Can you work these out from the model? Positions are in its coordinate system, mm. Round coordinates to 2 decimals unless told otherwise and drop trailing zeros. Loops run counter-clockwise (first coordinate to the right, second up) from the corner with the lowest first, then second, coordinate; pieces in that order, holes last.
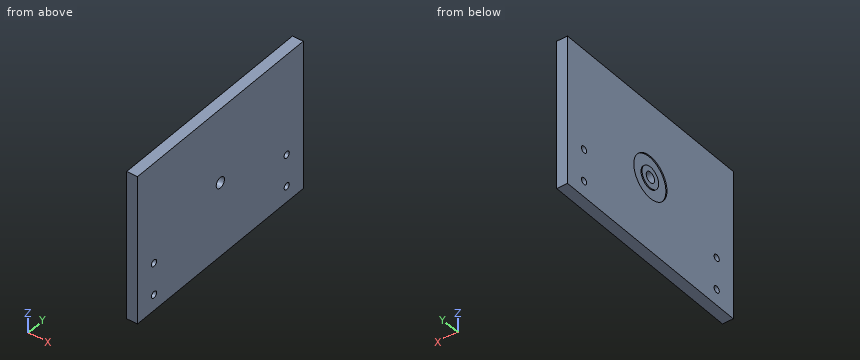
Solid Edge part; units mm, degrees
sketch "Sketch1" plane through (0, 0, 0) normal (1, 0, 0) x (0, 1, 0)
  line L0 (-80.5059, -20.8442) -> (119.4941, -20.8442)
  line L1 (119.4941, -20.8442) -> (119.4941, 119.1558)
  line L2 (119.4941, 119.1558) -> (-80.5059, 119.1558)
  line L3 (-80.5059, 119.1558) -> (-80.5059, -20.8442)
  dimension "D1" = 80.5059
  dimension "D2" = 80.5059
extrude "Protrusion1" add sketch "Sketch1" against normal blind 10
sketch "Sketch2" plane through (0, 44.4941, 29.1558) normal (1, 0, 0) x (0, 1, 0)
  circle A0 centre (-25, 20) radius 5
extrude "Cutout1" cut sketch "Sketch2" against normal through all
sketch "Sketch3" plane through (-10, 44.4941, 29.1558) normal (-1, 0, 0) x (0, -1, 0)
  circle A0 centre (25, 20) radius 10
  circle A1 centre (25, 20) radius 20
extrude "Cutout2" cut sketch "Sketch3" against normal blind 1
hole "Hole1" at (-10, 99.4941, -5.8442) direction (1, 0, 0) diameter 6.2 end up to next
hole "Hole2" at (-10, -60.5059, -5.8442) direction (1, 0, 0) diameter 6.2 end up to next
hole "Hole3" at (-10, -60.5059, 24.1558) direction (1, 0, 0) diameter 6.2 end up to next
hole "Hole4" at (-10, 99.4941, 24.1558) direction (1, 0, 0) diameter 6.2 end up to next
(1) If I drill on line 1 (Z direction, x = -0.75, y = -59); line 2 (X direction, y = 36.5, z = 40); line 3 (Y direction, x = -6.75, z = 21.5), over which ranges is the centre line in solid material (lowest first)?
Worked answers:
line 1: z = -20.84 to -8.55, -3.13 to 21.45, 26.87 to 119.16
line 2: x = -9 to 0
line 3: y = -80.51 to -62.1, -58.91 to 97.9, 101.09 to 119.49
(2) If we section it at B-B, the plane y = 7: List the corners of the cut face in (x, z) for me.
Worked answers:
outline: (-10, -20.84) - (0, -20.84) - (0, 119.16) - (-10, 119.16) - (-10, 64.77) - (-9, 64.77) - (-9, 33.54) - (-10, 33.54) - close
(3) If we section it at C-C, the plane y = 34: List the corners of the cut face in (x, z) for me, then the cut area to 3 significant figures.
Worked answers:
outline: (-10, -20.84) - (0, -20.84) - (0, 119.16) - (-10, 119.16) - (-10, 62.92) - (-9, 62.92) - (-9, 35.39) - (-10, 35.39) - close
area: 1,370 mm2
(4) If we section it at A-A, the plane z = 52: List the corners of the cut face in (x, y) for me.
Worked answers:
outline: (-10, -80.51) - (0, -80.51) - (0, 15.38) - (-10, 15.38) - (-10, 9.91) - (-9, 9.91) - (-9, -0.3) - (-10, -0.3) - close; (-10, 23.61) - (0, 23.61) - (0, 119.49) - (-10, 119.49) - (-10, 39.29) - (-9, 39.29) - (-9, 29.08) - (-10, 29.08) - close
(5) Will this pin go through, and if not, where does the flat tip stop? P1, Ø6, axis at y = 19.49, z = 49.16, coming from the -X side.
Worked answers:
P1: passes through
